Can you work these out from the model? Positions are in its coordinate system, mm. A direction names the side the tool comes from. Coordinates: 2 decimals unless noted, no trailing zeros. Order: outer loops, then holes, each group sorted by start corner. A loop starts at its lowest first (then second) coordinate and runs counter-clockwise, first axis right, second up. Notation, with made-up numbers: (10, 39) - (33, 39) arc R23 cw to (33, 70) - close; hole circle Ø10 at (-11.5, -25). An arc over 180 degrees is marked (long way). Use a Markdown table: item, result. Add a question column.
(1) We'd pull the mould along X, two halves only. Please class faces 4 (the flat face through (7.5, 6, 4)), 5 (the flat face through (-1.334, 30.018, 1.646)), 6 (the flat face through (-3, 3, 0)): pulls with the +X half, pulls with the -X half, needs draft (parallel to the pull), parting line crosses it, or undercut.
(2) I want a section at A-A (y = 14). List the corners of the cut face in (x, z) for me.
(3) I want a section at D-D (x = 5.25). List the corners of the cut face in (y, z) for me, and give its area (3 significant figures).
(4) For pin 1 Ø1.5 at (x, y) = (0, -7) entering from +Z; pin 2 Ø1.8 at (x, z) = (0, 4) entering from +Y, each with a flat end and sliding along its axis, tell me the tip position at first contact or that it passes through.
(5) I want a section at B-B (z = 6.5). List the corners of the cut face in (x, y) for me (3 decimals).
(6) On a 3-axis mill with a long thin cutter (end or side, diameter ignored), from which of +Z, -Z, +X, -X, +Y, -Y can I reach the whole of each face in a straight line? I mean faces 1 (the flat face through (0, 28.75, 6)), 2 (the cylindrical face through (0.1, -24.5, 3.9)), 3 (the cylindrical face through (1.487, 26.408, 3.805)). Say none if no direction works.
(7) If I drill on L1, parallel to Y at x = -0.25, z = 7; L2, parallel to X at y = 32.95, z = 4; L3, parallel to X at y = -19.5, z = 0.5, over which ranges is the centre line in solid material (lowest first)? Write a range as [from, to].
(8) I want a section at C-C (z = 4). List the corners of the cut face in (x, y) for me (3 decimals), and give its area (3 significant figures).
```python
from build123d import *

# Parameters (mm, degrees)
BOSS_EXTRUDE1_DEPTH     = 8
CUT_EXTRUDE2_START      = -2.5
CUT_EXTRUDE2_DEPTH      = 2.5
SKETCH4_W               = 5.41
SKETCH4_H               = 2.5
CUT_EXTRUDE3_DEPTH      = 4
CUT_EXTRUDE4_REACH      = 66.194
CUT_EXTRUDE4_END_RADIUS = 2.5
SKETCH5_R               = 1.5


with BuildPart() as part:
    # Sketch1 → Boss-Extrude1 (new body)
    with BuildSketch(Plane.XY):
        with BuildLine():
            Line((-7.5, 33.75), (7.5, 33.75))
            Line((7.5, 33.75), (7.5, -22))
            ThreePointArc((7.5, -22), (0, -29.5), (-7.5, -22))
            Line((-7.5, -22), (-7.5, 33.75))
        make_face()
        with BuildLine():
            Line((2.5, 22), (2.5, -22))
            ThreePointArc((2.5, -22), (0, -24.5), (-2.5, -22))
            Line((-2.5, -22), (-2.5, 22))
            ThreePointArc((-2.5, 22), (0, 24.5), (2.5, 22))
        make_face(mode=Mode.SUBTRACT)
    extrude(amount=BOSS_EXTRUDE1_DEPTH)

    # Sketch3 → Cut-Extrude2 (cut)
    with BuildSketch(Plane(origin=(0, 33.75, 0), x_dir=(1, 0, 0), z_dir=(0, 1, 0)).offset(CUT_EXTRUDE2_START)):
        Polygon((0, -7.123464956), (2.705, -5.561732478), (2.705, -2.438267522), (0, -0.876535044), (-2.705, -2.438267522), (-2.705, -5.561732478), align=None)
    extrude(amount=-CUT_EXTRUDE2_DEPTH, mode=Mode.SUBTRACT)

    # Sketch4 → Cut-Extrude3 (cut)
    with BuildSketch(Plane.XY.offset(8)):
        with Locations((0, 30)):
            Rectangle(SKETCH4_W, SKETCH4_H)
    extrude(amount=-CUT_EXTRUDE3_DEPTH, mode=Mode.SUBTRACT)

    # Cut-Extrude4: up to this cylinder (the profile starts outside it)
    cut_extrude4_end = Plane(origin=(0, 22, 4), z_dir=(0, 0, -1)) * Cylinder(CUT_EXTRUDE4_END_RADIUS, 138.388, mode=Mode.PRIVATE)
    # Sketch5 → Cut-Extrude4 (cut, up to the surface)
    with BuildSketch(Plane(origin=(0, 33.75, 0), x_dir=(1, 0, 0), z_dir=(0, 1, 0)), mode=Mode.PRIVATE) as cut_extrude4_sk1:
        with Locations(Location((0, -4, 0), (0, 0, 270))):
            Circle(SKETCH5_R)
    cut_extrude4_tool1 = extrude(cut_extrude4_sk1.sketch, amount=-CUT_EXTRUDE4_REACH, mode=Mode.PRIVATE) - cut_extrude4_end
    add(cut_extrude4_tool1.solids().sort_by_distance((0, 33.75, 4))[0], mode=Mode.SUBTRACT)


solid = part.part
```
Answers follow:
| question | item | result |
|---|---|---|
| 1 | face 4 | pulls with the +X half |
| 1 | face 5 | undercut |
| 1 | face 6 | needs draft |
| 2 | outline | (-7.5, 0) - (-2.5, 0) - (-2.5, 8) - (-7.5, 8) - close; (2.5, 0) - (7.5, 0) - (7.5, 8) - (2.5, 8) - close |
| 3 | outline | (-27.36, 0) - (33.75, 0) - (33.75, 8) - (-27.36, 8) - close |
| 3 | area | 489 mm² |
| 4 | pin 1 | passes through |
| 4 | pin 2 | stops at y = -24.33 |
| 5 | outline | (-7.5, -22) arc R7.5 ccw to (7.5, -22) - (7.5, 33.75) - (-7.5, 33.75) - close; hole (-2.705, 28.75) - (2.705, 28.75) - (2.705, 31.25) - (-2.705, 31.25) - close; hole (-2.5, -22) arc R2.5 ccw to (2.5, -22) - (2.5, 22) arc R2.5 ccw to (-2.5, 22) - close |
| 6 | face 1 | +Z |
| 6 | face 2 | +Z, -Z |
| 6 | face 3 | +Y |
| 7 | L1 | y = [-29.5, -24.49], [24.49, 28.75], [31.25, 33.75] |
| 7 | L2 | x = [-7.5, -1.5], [1.5, 7.5] |
| 7 | L3 | x = [-7.5, -2.5], [2.5, 7.5] |
| 8 | outline | (-7.5, -22) arc R7.5 ccw to (7.5, -22) - (7.5, 33.75) - (1.5, 33.75) - (1.5, 31.25) - (2.705, 31.25) - (2.705, 28.75) - (1.5, 28.75) - (1.5, 24) arc R2.5 cw to (2.5, 22) - (2.5, -22) arc R2.5 cw to (-2.5, -22) - (-2.5, 22) arc R2.5 cw to (-1.5, 24) - (-1.5, 28.75) - (-2.705, 28.75) - (-2.705, 31.25) - (-1.5, 31.25) - (-1.5, 33.75) - (-7.5, 33.75) - close |
| 8 | area | 651 mm² |
